Here's how the part is built. I have some questions about the finished solid (model axes, mm). A direction names the side the tool comes from. Coordinates: 2 decimals unless noted, no trailing zeros. Write each loop counter-clockwise with the first axis right and the second up, starting at its lowest first coordinate (ties: lowest second). Pieces come first, ordered by that corner, then holes. Notation, with made-up numbers: (55.5, 63.5) -> (60.5, 63.5) arc R29 cw to (60.5, 88.5) -> close; hole circle Ø3 at (-23, -23.75). An arc over 180 degrees is marked (long way). Put each result on its own line as item: value. Start each with the question number.
Item 1: If we mould it in two halves opening along Z, with no side actions, what happens to faces 3 (the face through (0, 1, -16)), 4 (the face through (4.93, 74.362, 9.764)), 5 (the face through (3, -1.3, 21.3)), 6 (the face through (1, 0, -6))? For each: released by +Z, released by -Z, zero draft, split by the parting line, or undercut.
Item 2: I want a section at C-C, the plane y = 20. List the corners of the cut face in (x, z) for me.
Item 3: I want a section at A-A, the plane z = 0. List the corners of the cut face in (x, y) for me, then the cut area to 3 significant figures.
Item 4: For pin 1 (3.5 mm diameter, centred on y = 0, z = 0, fed in from +X); pin 2 (3 mm diameter, centred on y = -1, z = 19, fed in from -X); pin 3 (2 mm diameter, centred on x = 6, y = -58, fed in from +Z); pin 4 (1 mm diameter, centred on x = 4.5, y = 41, fed in from +Z), each with a flat end and sliding along its axis, tell me the tip position at first contact or that it passes through.
Item 5: I need wall thicknesses on line 1 (Z direction, x = 6.25, y = 1); line 2 (Y direction, x = 2.35, z = 0); line 3 (Y direction, x = 1.4, z = -20). Which ranges of each line are inside material? Lowest first, please. Write a range as [from, to].
Item 6: I want a section at B-B, the plane x = 1.5. List the corners of the cut face in (y, z) for me.
Item 7: On a 3-axis mill with a long thin cutter (end or side, diameter ignored), from which of +Z, -Z, +X, -X, +Y, -Y can I reach the whole of each face in a straight line? I mean faces 1 (the face through (1, 0, 17)), 2 (the face through (10, 1, -16)). Say none if no direction works.
Item 8: I want a section at D-D, the plane z = -61. List the corners of the cut face in (x, y) for me, then the cut area to 3 significant figures.
from build123d import *

# Parameters (mm, degrees)
SKETCH_1_R          = 75
EXTRUDE_1_DEPTH     = 10
SKETCH_2_R          = 3
SKETCH_2_R_2        = 1.5
CUT_EXTRUDE_1_DEPTH = 10
SKETCH_3_R          = 6
CUT_EXTRUDE_2_DEPTH = 3
SKETCH_4_R          = 3
CUT_EXTRUDE_3_DEPTH = 3
SKETCH_5_R          = 3
CUT_EXTRUDE_4_DEPTH = 3


with BuildPart() as part:
    # 草图1 → 凸台-拉伸1 (new body)
    with BuildSketch(Plane(origin=(0, 0, 0), x_dir=(0, 0, -1), z_dir=(1, 0, 0))):
        Circle(SKETCH_1_R)
    extrude(amount=EXTRUDE_1_DEPTH)

    # 草图2 → 切除-拉伸1 (cut)
    with BuildSketch(Plane(origin=(10, 0, 0), x_dir=(0, 0, -1), z_dir=(1, 0, 0))):
        Circle(SKETCH_2_R)
        with Locations((-20, 0)):
            Circle(SKETCH_2_R_2)
        with Locations((20, 0)):
            Circle(SKETCH_2_R_2)
    extrude(amount=-CUT_EXTRUDE_1_DEPTH, mode=Mode.SUBTRACT)

    # 草图3 → 切除-拉伸2 (cut)
    with BuildSketch(Plane.ZY):
        Circle(SKETCH_3_R)
    extrude(amount=-CUT_EXTRUDE_2_DEPTH, mode=Mode.SUBTRACT)

    # 草图4 → 切除-拉伸3 (cut)
    with BuildSketch(Plane.ZY):
        with Locations((20, 0)):
            Circle(SKETCH_4_R)
    extrude(amount=-CUT_EXTRUDE_3_DEPTH, mode=Mode.SUBTRACT)

    # 草图5 → 切除-拉伸4 (cut)
    with BuildSketch(Plane.ZY):
        with Locations((-20, 0)):
            Circle(SKETCH_5_R)
    extrude(amount=-CUT_EXTRUDE_4_DEPTH, mode=Mode.SUBTRACT)


solid = part.part
Calculated:
1. face 3: zero draft
1. face 4: split by the parting line
1. face 5: undercut
1. face 6: undercut
2. outline: (0, -72.28) -> (10, -72.28) -> (10, 72.28) -> (0, 72.28) -> close
3. outline: (0, -75) -> (10, -75) -> (10, -3) -> (3, -3) -> (3, -6) -> (0, -6) -> close; (0, 6) -> (3, 6) -> (3, 3) -> (10, 3) -> (10, 75) -> (0, 75) -> close
3. area: 1,420 mm2
4. pin 1: passes through
4. pin 2: stops at x = 3
4. pin 3: stops at z = 48.74
4. pin 4: stops at z = 63.12
5. line 1: z = [-74.99, -21.12], [-18.88, -2.83], [2.83, 18.88], [21.12, 74.99]
5. line 2: y = [-75, -6], [6, 75]
5. line 3: y = [-72.28, -3], [3, 72.28]
6. outline: circle Ø150 at (0, 0); hole circle Ø12 at (0, 0); hole circle Ø6 at (0, -20); hole circle Ø6 at (0, 20)
7. face 1: -X
7. face 2: +Z, -Z, +X, +Y, -Y
8. outline: (0, -43.63) -> (10, -43.63) -> (10, 43.63) -> (0, 43.63) -> close
8. area: 873 mm2
